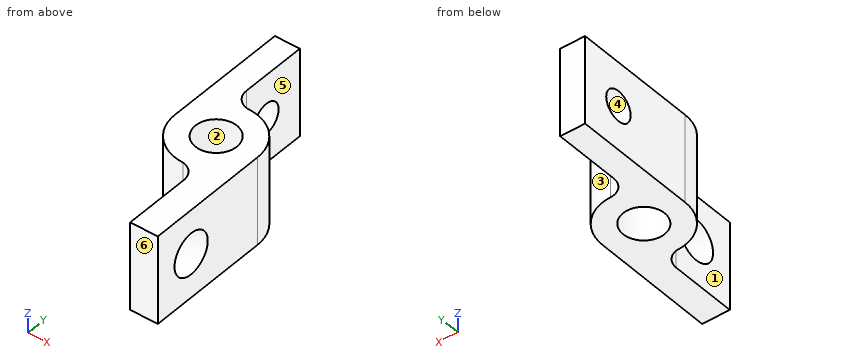
Autodesk Inventor part; units mm, degrees
ref_plane "YZ Plane" through (0, 0, 0) normal (1, 0, 0) x (0, 1, 0)
ref_plane "XZ Plane" through (0, 0, 0) normal (0, 1, 0) x (-1, 0, 0)
ref_plane "XY Plane" through (0, 0, 0) normal (0, 0, 1) x (1, 0, 0)
sketch "Náčrt1" plane through (0, 0, 0) normal (0, 0, 1) x (1, 0, 0)
  line L0 (5.1631, -20.9413) -> (5.1631, -45)
  arc A0 (5.1631, -20.9413) -> (0, -15) centre (-0.8369, -20.9413) ccw
  line L1 (5.1631, -45) -> (15.1631, -45)
  line L2 (15.1631, -45) -> (14.9999, 0.0543)
  line L3 (-14.9999, 0.0543) -> (-14.9999, 45)
  arc A1 (-6, 21) -> (0, 15) centre (0, 21) ccw
  line L4 (-6, 21) -> (-6, 45)
  line L5 (-6, 45) -> (-14.9999, 45)
  circle A2 centre (0, 0) radius 7.5
  arc A3 (-14.9999, 0.0543) -> (0, -15) centre (0, 0) ccw
  arc A4 (14.9999, 0.0543) -> (0, 15) centre (0, 0) ccw
  dimension "d1" = 6
  dimension "d2" = 45
  dimension "d3" = 10
  dimension "d10" = 12
  dimension "d11" = 15
extrude "Vysunutí1" add sketch "Náčrt1" along normal blind 32
sketch "Náčrt2" plane through (14.9999, 0.0543, 32) normal (1, 0.0036, 0) x (0, 0, -1)
  line L0 (32, -45.0184) -> (0, -45.0184)
  circle A0 centre (16, -30.0184) radius 7.5
  line L1 (32, -45.0546) -> (32, 0)
  dimension "d15" = 15
  dimension "d16" = 15
  dimension "d17" = 16
extrude "Vysunutí2" cut sketch "Náčrt2" against normal blind 32
sketch "Náčrt3" plane through (-6, 21, 0) normal (1, 0, 0) x (0, 0, -1)
  circle A0 centre (-16, 9) radius 5.4921
  line L0 (0, 0) -> (0, 24)
  line L1 (0, 24) -> (-32, 24)
  point P0 (0, -21)
  dimension "d20" = 16
  dimension "d21" = 15
extrude "Vysunutí3" cut sketch "Náčrt3" against normal blind 32
properties part number "15"
Can you work these out from the model? Positions are in its coordinate system, mm. Face numbers are marked on the shaded views. A direction names the side the tool comes from. Round coordinates to 2 decimals unless told otherwise and drop trailing zeros. Order: outer loops, then holes, each group sorted by start corner. A loop starts at its lowest first (then second) coordinate and runs counter-clockwise, first axis right, second up. Notation, with made-up numbers: (59.5, 28) -> (90.5, 28) arc R15 cw to (90.5, 46) -> close; hole circle Ø10 at (57, 47). An arc over 180 degrees is marked (long way). Return JSON: item names as keys, results as strings. Group by question number.
1. I need wall thicknesses on line 1 (Y direction, x = 0, z = 17); line 2 (Y direction, x = -13, z = 16); line 3 (X direction, y = 39.5, z = 9.5). Which ranges of each line are inside material? Lowest first, please. Write a range as [from, to].
2. Which directions (+Z, -Z, +X, -X, +Y, -Y) give clear straight access to the entire face, cutting with the end or side of a thin tool? Please do the marked faces 5 and 6.
3. Will these pins go through, and if not, where does the flat tip stop? pin 1 (5 mm diameter, centred on x = 0.5, z = 15.5, fed in from +Y); pin 2 (6 mm diameter, centred on y = 34, z = 8.5, fed in from +X); pin 3 (17.5 mm diameter, centred on y = 30, z = 16, fed in from -X); pin 4 (2 mm diameter, centred on x = -0.5, z = 8, fed in from -Y).
4. If we section it at B-B, the plane y = 30: Write out the boundary of the cut face in (x, z).
5. If we section it at D-D, the plane x = -11: Write out the boundary of the cut face in (y, z), then the cut area to 3 significant figures.
6. If we section it at A-A, the plane z = 14: Write out the boundary of the cut face in (x, y) (3 decimals), then the cut area to 3 significant figures.
7. We'd pull the mould along X, two halves only. Please class the marked faces 1, 2, 3 and 4: released by +X, released by -X, zero draft, split by the parting line, or undercut.
8. If we section it at C-C, the plane z = 3.5: Write out the boundary of the cut face in (x, y), then the cut area to 3 significant figures.
Output values:
{
 "1": {"line 1": "[-15, -7.5], [7.5, 15]", "line 2": "[-7.48, 24.51], [35.49, 45]", "line 3": "[-15, -6]"},
 "2": {"face 5": "+Z, -Z, +X, +Y", "face 6": "+Z, -Z, +X, -X, -Y"},
 "3": {"pin 1": "y = 15.34", "pin 2": "x = -6", "pin 3": "x = -15", "pin 4": "y = -15.09"},
 "4": {"outline": "(-15, 0) -> (-6, 0) -> (-6, 10.51) -> (-15, 10.51) -> close; (-15, 21.49) -> (-6, 21.49) -> (-6, 32) -> (-15, 32) -> close"},
 "5": {"outline": "(-10.2, 0) -> (45, 0) -> (45, 32) -> (-10.2, 32) -> close; hole circle Ø10.98 at (30, 16)", "area": "1,670 mm²"},
 "6": {"outline": "(-15, 0.054) arc R15 ccw to (0, -15) arc R6 cw to (5.163, -20.941) -> (5.163, -22.771) -> (15.082, -22.736) -> (15, 0.054) arc R15 ccw to (0, 15) arc R6 cw to (-6, 21) -> (-6, 24.885) -> (-15, 24.885) -> close; (-15, 35.115) -> (-6, 35.115) -> (-6, 45) -> (-15, 45) -> close; (5.163, -45) -> (15.163, -45) -> (15.135, -37.192) -> (5.163, -37.228) -> close; hole circle Ø15 at (0, 0)", "area": "975 mm²"},
 "7": {"face 1": "released by -X", "face 2": "undercut", "face 3": "released by +X", "face 4": "zero draft"},
 "8": {"outline": "(-15, 0.05) arc R15 ccw to (0, -15) arc R6 cw to (5.16, -20.94) -> (5.16, -45) -> (15.16, -45) -> (15, 0.05) arc R15 ccw to (0, 15) arc R6 cw to (-6, 21) -> (-6, 45) -> (-15, 45) -> close; hole circle Ø15 at (0, 0)", "area": "1,210 mm²"}
}
